The listing builds one solid part. Answer for the finished solid, in the listing's coordinates (mm). Give positions to 0.01 mm unless a question says otherwise; leave off trailing zeros. Write each loop counter-clockwise with the first axis right and the second up, starting at its lowest first coordinate (ties: lowest second). Pieces come first, ordered by that corner, then holes. Notation, with made-up numbers: (-8.75, 62) - (3.25, 62) arc R15 ccw to (3.25, 73) - close; hole circle Ø2 at (-14.5, 81.25). An arc over 180 degrees is marked (long way). One line per question, with ' | ' between items. Start each with the question number.
1. Find the intervals of material crossed by L1, parallel to X at y = 77.5, z = 0.3; L2, parallel to Y at x = 695, z = 1.7; L3, parallel to Y at x = 661, z = 1, in increasing order. Write a range as from..to.
2. Given P1, Ø1.3, axis at x = 321.5, z = 1, coming from the -Y side; P2, Ø0.8, axis at y = 26.5, z = 1.5, coming from the +X side; P3, Ø1.3, axis at y = 4, z = 1, coming from the -X side, each flat-ended and moving along its own axis, determine where each tip first touches the part or whether it passes through.
3. A cutting plane is placed at A-A (y = 129.5). Determine the outline of the cut face in (x, z).
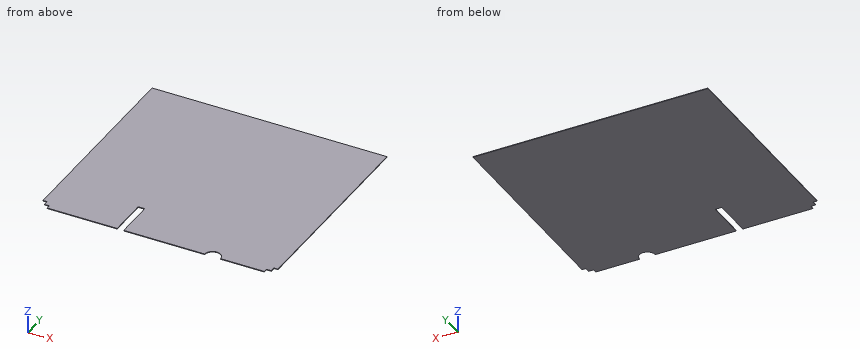
```python
from build123d import *

# Parameters (mm, degrees)
BOSS_EXTRUDE1_DEPTH = 2.54


with BuildPart() as part:
    # Sketch1 → Boss-Extrude1 (new body)
    with BuildSketch(Plane.XY):
        with BuildLine():
            Line((0, 825.5), (0, 34.544))
            Line((0, 34.544), (15.24, 34.544))
            Line((15.24, 34.544), (15.24, 15.24))
            Line((15.24, 15.24), (34.544, 15.24))
            Line((34.544, 15.24), (34.544, 0))
            Line((34.544, 0), (304.8, 0))
            Line((304.8, 0), (304.8, 152.4))
            Line((304.8, 152.4), (330.2, 152.4))
            Line((330.2, 152.4), (330.2, 0))
            Line((330.2, 0), (642.84098, 0))
            ThreePointArc((642.84098, 0), (673.32098, 30.48), (703.80098, 0))
            Line((703.80098, 0), (872.45698, 0))
            Line((872.45698, 0), (872.45698, 15.24))
            Line((872.45698, 15.24), (891.76098, 15.24))
            Line((891.76098, 15.24), (891.76098, 34.544))
            Line((891.76098, 34.544), (907.00098, 34.544))
            Line((907.00098, 34.544), (907.00098, 825.5))
            Line((907.00098, 825.5), (0, 825.5))
        make_face()
    extrude(amount=BOSS_EXTRUDE1_DEPTH)


solid = part.part
```
Determined:
1) L1: 0..304.8, 330.2..907 | L2: 21.43..825.5 | L3: 27.88..825.5
2) P1: y = 152.4 | P2: x = 891.76 | P3: x = 34.54
3) outline: (0, 0) - (304.8, 0) - (304.8, 2.54) - (0, 2.54) - close; (330.2, 0) - (907, 0) - (907, 2.54) - (330.2, 2.54) - close
